```python
from build123d import *

# Parameters (mm, degrees)
SKETCH1_W           = 200
SKETCH1_H           = 150
BOSS_EXTRUDE1_DEPTH = 5
SKETCH3_R           = 3
CUT_EXTRUDE2_DEPTH  = 10
FILLET1_R           = 20


with BuildPart() as part:
    # Sketch1 → Boss-Extrude1 (new body)
    with BuildSketch(Plane(origin=(0, 0, 0), x_dir=(1, 0, 0), z_dir=(0, 1, 0))):
        with Locations((15, 0)):
            Rectangle(SKETCH1_W, SKETCH1_H)
    extrude(amount=BOSS_EXTRUDE1_DEPTH)

    # Sketch3 → Cut-Extrude2 (cut)
    with BuildSketch(Plane(origin=(0, 5, 0), x_dir=(1, 0, 0), z_dir=(0, 1, 0))):
        with Locations(Location((-70, -43, 0), (0, 0, 270))):
            Circle(SKETCH3_R)
        with Locations(Location((-50, -43, 0), (0, 0, 270))):
            Circle(SKETCH3_R)
        with Locations(Location((0, -43, 0), (0, 0, 270))):
            Circle(SKETCH3_R)
        with Locations(Location((20, -43, 0), (0, 0, 270))):
            Circle(SKETCH3_R)
        with Locations(Location((-25, 20, 0), (0, 0, 270))):
            Circle(SKETCH3_R)
        with Locations(Location((-25, 34, 0), (0, 0, 270))):
            Circle(SKETCH3_R)
        with Locations(Location((95, 20, 0), (0, 0, 270))):
            Circle(SKETCH3_R)
        with Locations(Location((95, 34, 0), (0, 0, 270))):
            Circle(SKETCH3_R)
        with BuildLine():
            Line((40, -5), (55, -5))
            ThreePointArc((55, -5), (62.071067812, -2.071067812), (65, 5))
            Line((65, 5), (65, 55))
            ThreePointArc((65, 55), (62.071067812, 62.071067812), (55, 65))
            Line((55, 65), (40, 65))
            ThreePointArc((40, 65), (32.928932188, 62.071067812), (30, 55))
            Line((30, 55), (30, 5))
            ThreePointArc((30, 5), (32.928932188, -2.071067812), (40, -5))
        make_face()
        with BuildLine():
            Line((-60, -30), (-50, -30))
            ThreePointArc((-50, -30), (-42.928932188, -27.071067812), (-40, -20))
            Line((-40, -20), (-40, -5))
            ThreePointArc((-40, -5), (-42.928932188, 2.071067812), (-50, 5))
            Line((-50, 5), (-60, 5))
            ThreePointArc((-60, 5), (-67.071067812, 2.071067812), (-70, -5))
            Line((-70, -5), (-70, -20))
            ThreePointArc((-70, -20), (-67.071067812, -27.071067812), (-60, -30))
        make_face()
    extrude(amount=-CUT_EXTRUDE2_DEPTH, mode=Mode.SUBTRACT)

    # Fillet1
    fillet1_edges = [part.edges().sort_by_distance(p)[0] for p in [
        (-85, 2.5, -75),
        (115, 2.5, -75),
        (115, 2.5, 75),
        (-85, 2.5, 75),
    ]]
    fillet(fillet1_edges, radius=FILLET1_R)


solid = part.part
```
Part model, mm, in its own coordinate system. A direction names the side the tool comes from. Coordinates: 2 decimals unless noted, no trailing zeros. Write each loop counter-clockwise with the first axis right and the second up, starting at its lowest first coordinate (ties: lowest second). Pieces come first, ordered by that corner, then holes.
Item 1: Probe line 1 (X direction, y = 1.5, z = 43); line 2 (X direction, y = 2.55, z = -34); line 3 (Z direction, x = 43.5, y = 4.1). List the from-to ranges inside material, lowest first.
Item 2: Slice it at B-B (x = 20). Write the cut outline in (y, z), and give its area (3 significant figures).
Item 3: Slice it at D-D (y = 2.9). Count the separate pieces of the cut face and the enclosed holes in it, and give its area (3 significant figures).
Item 4: Slice it at A-A (z = -34). Write the cut outline in (x, y).
Item 5: Mould opens along X. For faces 1 (the face through (-25, 3, -37)), 2 (the face through (14, 2, 75)), 3 (the face through (115, 2, 1)) say: released by +X, released by -X, zero draft, split by the parting line, or undercut.
Item 6: Which spindle directions (+Z, -Z, +X, -X, +Y, -Y) get a long thin tool onto all of the face, cutting with end or side? Do faces 4 (the face through (14, 5, -1)), 5 (the face through (30, 3, -30)). Say none if no direction does.
Item 7: Slice it at C-C (z = 15.5). Write the cut outline in (x, y), and give its area (3 significant figures).
Results found:
1. line 1: x = -85 to -73, -67 to -53, -47 to -3, 3 to 17, 23 to 115
1. line 2: x = -85 to -28, -22 to 30, 65 to 92, 98 to 115
1. line 3: z = -75 to -65, 5 to 75
2. outline: (0, -75) - (5, -75) - (5, 40) - (0, 40) - close; (0, 46) - (5, 46) - (5, 75) - (0, 75) - close
2. area: 720 mm2
3. separate pieces: 1
3. enclosed holes: 10
3. area: 26,100 mm2
4. outline: (-85, 0) - (-28, 0) - (-28, 5) - (-85, 5) - close; (-22, 0) - (30, 0) - (30, 5) - (-22, 5) - close; (65, 0) - (92, 0) - (92, 5) - (65, 5) - close; (98, 0) - (115, 0) - (115, 5) - (98, 5) - close
5. face 1: undercut
5. face 2: zero draft
5. face 3: released by +X
6. face 4: +Z, -Z, +X, -X, +Y
6. face 5: +Y, -Y
7. outline: (-85, 0) - (-70, 0) - (-70, 5) - (-85, 5) - close; (-40, 0) - (115, 0) - (115, 5) - (-40, 5) - close
7. area: 850 mm2
